Autodesk Inventor part; units mm, degrees
ref_plane "YZ Plane" through (0, 0, 0) normal (1, 0, 0) x (0, 1, 0)
ref_plane "XZ Plane" through (0, 0, 0) normal (0, 1, 0) x (-1, 0, 0)
ref_plane "XY Plane" through (0, 0, 0) normal (0, 0, 1) x (1, 0, 0)
sketch "Sketch1" plane through (0, 0, 0) normal (0, 0, 1) x (1, 0, 0)
  line L0 (-15.8942, -5.4427) -> (36.1058, -5.4427)
  line L1 (36.1058, -5.4427) -> (36.1058, -0.4427)
  line L2 (36.1058, -0.4427) -> (50.1058, -0.4427)
  line L3 (50.1058, -0.4427) -> (50.1058, -5.4427)
  line L4 (50.1058, -5.4427) -> (82.1058, -5.4427)
  line L5 (82.1058, -5.4427) -> (82.1058, 41.5573)
  line L6 (82.1058, 41.5573) -> (47.1058, 41.5573)
  line L7 (47.1058, 41.5573) -> (47.1058, 57.5573)
  line L8 (47.1058, 57.5573) -> (13.1058, 57.5573)
  line L9 (13.1058, 57.5573) -> (-15.8942, 57.5573)
  line L10 (-15.8942, 57.5573) -> (-15.8942, -5.4427)
  point P0 (0, 0)
  dimension "d0" = 52
  dimension "d1" = 5
  dimension "d2" = 14
  dimension "d3" = 5
  dimension "d4" = 32
  dimension "d5" = 47
  dimension "d6" = 35
  dimension "d7" = 16
  dimension "d8" = 34
  dimension "d9" = 29
extrude "Extrusion1" add sketch "Sketch1" along normal blind 41
sketch "Sketch10" plane through (0, 0, 41) normal (0, 0, 1) x (1, 0, 0)
  line L0 (-15.8942, 57.5573) -> (-15.8942, -5.4427)
  line L1 (47.1058, 57.5573) -> (-15.8942, 57.5573)
  point P0 (0, 0)
  point P1 (13.569, 57.5573)
  dimension "d16" = 29.4632
sketch "Sketch12" plane through (0, 0, 41) normal (0, 0, 1) x (1, 0, 0)
  circle A0 centre (-80.4891, 35.6187) radius 25
  line L0 (47.1058, 57.5573) -> (-15.8942, 57.5573)
  circle A1 centre (13.4877, 29.5573) radius 25
  point P0 (0, 0)
  dimension "d17" = 50
  dimension "d18" = 50
  dimension "d19" = 28
extrude "Extrusion2" cut sketch "Sketch12" against normal blind 13 contours A1
sketch "Sketch13" plane through (0, 0, 41) normal (0, 0, 1) x (1, 0, 0)
  circle A0 centre (-18.8292, 31.3442) radius 32
  circle A1 centre (13.4877, 29.5573) radius 25
  line L0 (13.4877, 54.5573) -> (13.4877, 4.5573)
  circle A2 centre (-13.4781, 30.9626) radius 27
  point P0 (0, 0)
  dimension "d22" = 64
  dimension "d23" = 54
extrude "Extrusion3" cut sketch "Sketch13" against normal through all contours A0 A2 A1 | A0 A2 L0 | A2 L0 | A1 A2 picked at (-3.1402, 31.014)
sketch "Sketch14" plane through (0, 0, 41) normal (0, 0, 1) x (1, 0, 0)
  arc A0 (0.7748, 8.031) -> (3.0811, 52.2884) centre (-13.4781, 30.9626) ccw
  line L0 (13.5219, 30.9626) -> (13.5219, 57.5526)
  line L1 (13.5219, 57.5526) -> (-18.1655, 57.5526)
  line L2 (-18.1655, 57.5526) -> (13.5219, 30.9626)
  point P0 (0, 0)
  dimension "d26" = 41.3657
  dimension "d27" = 31.6874
extrude "Extrusion4" cut sketch "Sketch14" against normal through all
sketch "Sketch15" plane through (0, 0, 41) normal (0, 0, 1) x (1, 0, 0)
  point P0 (0, 0)
sketch "Sketch16" plane through (0, 0, 0) normal (0, 0, -1) x (-1, 0, 0)
  circle A0 centre (18.3913, 30.8453) radius 32
  point P0 (0, 0)
  dimension "d30" = 64
extrude "Extrusion5" cut sketch "Sketch16" against normal blind 33
sketch "Sketch21" plane through (47.1058, 57.5573, 41) normal (0, 1, 0) x (1, 0, 0)
  line L0 (0, 41) -> (-47.877, 41)
  line L1 (-63, 8) -> (-63, 41)
  point P0 (-47.1058, 41)
  point P1 (-25, 25)
  dimension "d33" = 16
  dimension "d34" = 38
hole "Hole1" at (22.1058, 57.5573, 16) direction (0, -1, 0) diameter 9.376 depth 29.3 tip angle 118
sketch "Sketch22" plane through (47.1058, 57.5573, 41) normal (0, 1, 0) x (1, 0, 0)
  point P0 (-47.1058, 41)
Verification items for the finished model (mm, model axes). A direction names the side the tool comes from. Give positions to 0.01 mm unless a question says otherwise; leave off trailing zeros. Loops run counter-clockwise (first coordinate to the right, second up) from the corner with the lowest first, then second, coordinate; pieces in that order, holes last. Notation, with made-up numbers: (29.5, 1.5) - (64.5, 1.5) arc R17 cw to (64.5, 27.5) - close; hole circle Ø2 at (49.5, 4.25). An arc over 180 degrees is marked (long way). Write item = value, one per line. Start each with the question number.
Q1. Thickness scan on line 1 (X direction, y = 49.25, z = 16); line 2 (X direction, y = 34, z = 16); line 3 (Y direction, x = 62, z = 23). Record the ranges inside material, lowest first.
Q2. Cross-section at D-D, the plane x = 75. Enter the section's corners in (y, z).
Q3. Mould release check, pull along Y, two halves, no side actions. Record for faces 1 (the face through (66, -5.443, 20)), 2 (the face through (65, 41.557, 20)), 3 (the face through (24, 24, 28)): released by +Y, released by -Y, zero draft, split by the parting line, or undercut.
Q4. Cross-section at B-B, the plane y = 44. Enter the section's corners in (x, z), and give its area (3 significant figures).
Q5. Tool access check on faces 4 (the face through (24.96, 42.7, 12.28)), 5 (the face through (47.106, 49, 20)), 6 (the face through (43, -0.443, 20)), 7 (the face through (13.522, 45, 16)), 8 (the face through (37.42, 22.33, 34.59)). Record the directions out of +Z, -Z, +X, -X, +Y, -Y that give a thin tool (end or side, any length) a straight path to the whole face; none if there is none.
Q6. Depth check by flat-ended pin: P1, Ø12, axis at x = 22.11, z = 16, coming from the +Y side; P2, Ø3, axis at x = 4, y = 8.5, coming from the +Z side; P3, Ø10, axis at y = 32.5, z = 17.5, coming from the -X side; P4, Ø3, axis at y = 11, z = 9, coming from the -X side. Enter the tip coordinate at first touch or a pass-through.
Answer key:
q1.line_1 = 13.52 to 17.42, 26.79 to 47.11
q1.line_2 = 13.52 to 17.42, 26.79 to 82.11
q1.line_3 = -5.44 to 41.56
q2.outline = (-5.44, 0) - (41.56, 0) - (41.56, 41) - (-5.44, 41) - close
q3.face_1 = released by -Y
q3.face_2 = released by +Y
q3.face_3 = undercut
q4.outline = (13.52, 0) - (47.11, 0) - (47.11, 41) - (33.89, 41) - (33.89, 28) - (13.52, 28) - close; hole circle Ø9.38 at (22.11, 16)
q4.area = 1,040 mm^2
q5.face_4 = +Y
q5.face_5 = +Z, -Z, +X, +Y
q5.face_6 = +Z, -Z, -Y
q5.face_7 = +Z, -Z, -X
q5.face_8 = +Z
q6.P1 = 57.56
q6.P2 = 28
q6.P3 = 13.43
q6.P4 = 5.45
